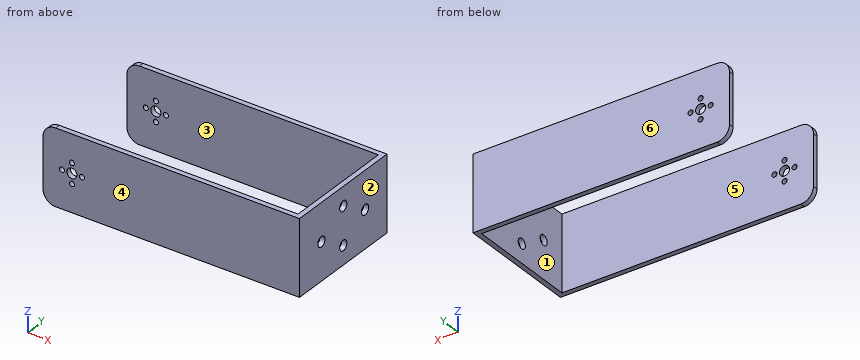
from build123d import *

# Parameters (mm, degrees)
EKSTR_ZYON_NCE1_DEPTH = 60
RADYUS1_R             = 10
KES_EKSTR_ZYON1_REACH = 236.137
IZIM2_R               = 4
IZIM2_R_2             = 2
KES_EKSTR_ZYON2_REACH = 234.491
IZIM3_R               = 4


with BuildPart() as part:
    # izim1 → Ekstr_zyon-_nce1 (new body)
    with BuildSketch(Plane.XY):
        Polygon((0, 0), (200, 0), (200, 90), (0, 90), (0, 94), (204, 94), (204, -4), (0, -4), align=None)
    extrude(amount=EKSTR_ZYON_NCE1_DEPTH)

    # Radyus1
    radyus1_edges = [part.edges().sort_by_distance(p)[0] for p in [
        (0, -2, 60),
        (0, 92, 60),
        (0, -2, 0),
        (0, 92, 0),
    ]]
    fillet(radyus1_edges, radius=RADYUS1_R)

    # izim2 → Kes-Ekstr_zyon1 (cut, up to next)
    with BuildSketch(Plane(origin=(0, 94, 0), x_dir=(1, 0, 0), z_dir=(0, 1, 0)), mode=Mode.PRIVATE) as kes_ekstr_zyon1_sk1:
        with Locations(Location((23, -30, 0), (0, 0, 270))):
            Circle(IZIM2_R)
    kes_ekstr_zyon1_tool1 = extrude(kes_ekstr_zyon1_sk1.sketch, amount=-KES_EKSTR_ZYON1_REACH, mode=Mode.PRIVATE) & part.part
    # izim2 → Kes-Ekstr_zyon1 (cut, up to next)
    with BuildSketch(Plane(origin=(0, 94, 0), x_dir=(1, 0, 0), z_dir=(0, 1, 0)), mode=Mode.PRIVATE) as kes_ekstr_zyon1_sk2:
        with Locations(Location((23, -22, 0), (0, 0, 270))):
            Circle(IZIM2_R_2)
    kes_ekstr_zyon1_tool2 = extrude(kes_ekstr_zyon1_sk2.sketch, amount=-KES_EKSTR_ZYON1_REACH, mode=Mode.PRIVATE) & part.part
    # izim2 → Kes-Ekstr_zyon1 (cut, up to next)
    with BuildSketch(Plane(origin=(0, 94, 0), x_dir=(1, 0, 0), z_dir=(0, 1, 0)), mode=Mode.PRIVATE) as kes_ekstr_zyon1_sk3:
        with Locations(Location((23, -38, 0), (0, 0, 270))):
            Circle(IZIM2_R_2)
    kes_ekstr_zyon1_tool3 = extrude(kes_ekstr_zyon1_sk3.sketch, amount=-KES_EKSTR_ZYON1_REACH, mode=Mode.PRIVATE) & part.part
    # izim2 → Kes-Ekstr_zyon1 (cut, up to next)
    with BuildSketch(Plane(origin=(0, 94, 0), x_dir=(1, 0, 0), z_dir=(0, 1, 0)), mode=Mode.PRIVATE) as kes_ekstr_zyon1_sk4:
        with Locations(Location((31, -30, 0), (0, 0, 270))):
            Circle(IZIM2_R_2)
    kes_ekstr_zyon1_tool4 = extrude(kes_ekstr_zyon1_sk4.sketch, amount=-KES_EKSTR_ZYON1_REACH, mode=Mode.PRIVATE) & part.part
    # izim2 → Kes-Ekstr_zyon1 (cut, up to next)
    with BuildSketch(Plane(origin=(0, 94, 0), x_dir=(1, 0, 0), z_dir=(0, 1, 0)), mode=Mode.PRIVATE) as kes_ekstr_zyon1_sk5:
        with Locations(Location((15, -30, 0), (0, 0, 270))):
            Circle(IZIM2_R_2)
    kes_ekstr_zyon1_tool5 = extrude(kes_ekstr_zyon1_sk5.sketch, amount=-KES_EKSTR_ZYON1_REACH, mode=Mode.PRIVATE) & part.part
    kes_ekstr_zyon1_1 = kes_ekstr_zyon1_tool1.solids().sort_by_distance((23, 94, 30))[0]
    add(kes_ekstr_zyon1_1, mode=Mode.SUBTRACT)
    kes_ekstr_zyon1_2 = kes_ekstr_zyon1_tool2.solids().sort_by_distance((23, 94, 22))[0]
    add(kes_ekstr_zyon1_2, mode=Mode.SUBTRACT)
    kes_ekstr_zyon1_3 = kes_ekstr_zyon1_tool3.solids().sort_by_distance((23, 94, 38))[0]
    add(kes_ekstr_zyon1_3, mode=Mode.SUBTRACT)
    kes_ekstr_zyon1_4 = kes_ekstr_zyon1_tool4.solids().sort_by_distance((31, 94, 30))[0]
    add(kes_ekstr_zyon1_4, mode=Mode.SUBTRACT)
    kes_ekstr_zyon1_5 = kes_ekstr_zyon1_tool5.solids().sort_by_distance((15, 94, 30))[0]
    add(kes_ekstr_zyon1_5, mode=Mode.SUBTRACT)
    kes_ekstr_zyon1 = kes_ekstr_zyon1_1 + kes_ekstr_zyon1_2 + kes_ekstr_zyon1_3 + kes_ekstr_zyon1_4 + kes_ekstr_zyon1_5  # Kes-Ekstr_zyon1 as one shape, for the pattern or mirror that repeats it

    # Aynalama1: Kes-Ekstr_zyon1 across plane
    add(kes_ekstr_zyon1.mirror(Plane.ZX.offset(45)), mode=Mode.SUBTRACT)

    # izim3 → Kes-Ekstr_zyon2 (cut, up to next)
    with BuildSketch(Plane(origin=(204, 0, 0), x_dir=(0, 0, -1), z_dir=(1, 0, 0)), mode=Mode.PRIVATE) as kes_ekstr_zyon2_sk1:
        with Locations((-30, 69.5)):
            Circle(IZIM3_R)
    kes_ekstr_zyon2_tool1 = extrude(kes_ekstr_zyon2_sk1.sketch, amount=-KES_EKSTR_ZYON2_REACH, mode=Mode.PRIVATE) & part.part
    # izim3 → Kes-Ekstr_zyon2 (cut, up to next)
    with BuildSketch(Plane(origin=(204, 0, 0), x_dir=(0, 0, -1), z_dir=(1, 0, 0)), mode=Mode.PRIVATE) as kes_ekstr_zyon2_sk2:
        with Locations((-45, 45)):
            Circle(IZIM3_R)
    kes_ekstr_zyon2_tool2 = extrude(kes_ekstr_zyon2_sk2.sketch, amount=-KES_EKSTR_ZYON2_REACH, mode=Mode.PRIVATE) & part.part
    # izim3 → Kes-Ekstr_zyon2 (cut, up to next)
    with BuildSketch(Plane(origin=(204, 0, 0), x_dir=(0, 0, -1), z_dir=(1, 0, 0)), mode=Mode.PRIVATE) as kes_ekstr_zyon2_sk3:
        with Locations(Location((-15, 45, 0), (0, 0, 180))):
            Circle(IZIM3_R)
    kes_ekstr_zyon2_tool3 = extrude(kes_ekstr_zyon2_sk3.sketch, amount=-KES_EKSTR_ZYON2_REACH, mode=Mode.PRIVATE) & part.part
    # izim3 → Kes-Ekstr_zyon2 (cut, up to next)
    with BuildSketch(Plane(origin=(204, 0, 0), x_dir=(0, 0, -1), z_dir=(1, 0, 0)), mode=Mode.PRIVATE) as kes_ekstr_zyon2_sk4:
        with Locations(Location((-30, 20.5, 0), (0, 0, 180))):
            Circle(IZIM3_R)
    kes_ekstr_zyon2_tool4 = extrude(kes_ekstr_zyon2_sk4.sketch, amount=-KES_EKSTR_ZYON2_REACH, mode=Mode.PRIVATE) & part.part
    add(kes_ekstr_zyon2_tool1.solids().sort_by_distance((204, 69.5, 30))[0], mode=Mode.SUBTRACT)
    add(kes_ekstr_zyon2_tool2.solids().sort_by_distance((204, 45, 45))[0], mode=Mode.SUBTRACT)
    add(kes_ekstr_zyon2_tool3.solids().sort_by_distance((204, 45, 15))[0], mode=Mode.SUBTRACT)
    add(kes_ekstr_zyon2_tool4.solids().sort_by_distance((204, 20.5, 30))[0], mode=Mode.SUBTRACT)


solid = part.part
Build history of the part. All positions in model axes, mm. Face numbers are marked on the shaded views. A direction names the side the tool comes from. Round coordinates to 2 decimals unless told otherwise and drop trailing zeros. Loops run counter-clockwise (first coordinate to the right, second up) from the corner with the lowest first, then second, coordinate; pieces in that order, holes last. Notation, with made-up numbers: (49.25, 4) -> (60.25, 4) arc R23 cw to (60.25, 13) -> close; hole circle Ø4 at (51.5, -30). An arc over 180 degrees is marked (long way). One line per item, written item: value. Start each with the question number.
Q1. Cut at A-A on z = 38. List the corners of the cut face in (x, y).
Q2. 3-axis set-ups, long thin cutter, end or side, ignore diameter. For the marked faces 1 and 2: which of +Z, -Z, +X, -X, +Y, -Y reach the whole face in a straight line?
Q3. Drop flat-ended pins along their axis: pin 1 Ø5 at (x, z) = (23, 38) entering from -Y; pin 2 Ø12 at (x, y) = (79, 7.5) entering from -Z; pin 3 Ø2 at (y, z) = (73.5, 46) entering from -X. Give the stop position or say it passes through.
Q4. Cut at B-B on x = 31. List the corners of the cut face in (y, z).
Q5. Probe line 1 along Y through (x, z) = (202.05, 30); line 2 along Y through (x, z) = (38, 52); line 3 along X through (y, z) = (-1.25, 22). List the from-to ranges inside material, lowest first.
Q6. Cut at C-C on y = 69.5. List the corners of the cut face in (x, z).
Q7. Cut at D-D on x = 70. List the corners of the cut face in (y, z).
Q8. Two-plate mould, pull along Y, no slides. Class the marked faces 3, 4, 5 and 6: released by +Y, released by -Y, zero draft, split by the parting line, or undercut.
Computed:
1. outline: (0, -4) -> (21, -4) -> (21, 0) -> (0, 0) -> close; (0, 90) -> (21, 90) -> (21, 94) -> (0, 94) -> close; (25, -4) -> (204, -4) -> (204, 94) -> (25, 94) -> (25, 90) -> (200, 90) -> (200, 0) -> (25, 0) -> close
2. face 1: +Z, -Z, -X
2. face 2: +Z, -Z, +X, +Y, -Y
3. pin 1: y = -4
3. pin 2: through
3. pin 3: x = 200
4. outline: (-4, 0) -> (0, 0) -> (0, 28) -> (-4, 28) -> close; (-4, 32) -> (0, 32) -> (0, 60) -> (-4, 60) -> close; (90, 0) -> (94, 0) -> (94, 28) -> (90, 28) -> close; (90, 32) -> (94, 32) -> (94, 60) -> (90, 60) -> close
5. line 1: -4 to 16.5, 24.5 to 65.5, 73.5 to 94
5. line 2: -4 to 0, 90 to 94
5. line 3: 0 to 21, 25 to 204
6. outline: (200, 0) -> (204, 0) -> (204, 26) -> (200, 26) -> close; (200, 34) -> (204, 34) -> (204, 60) -> (200, 60) -> close
7. outline: (-4, 0) -> (0, 0) -> (0, 60) -> (-4, 60) -> close; (90, 0) -> (94, 0) -> (94, 60) -> (90, 60) -> close
8. face 3: undercut
8. face 4: released by -Y
8. face 5: undercut
8. face 6: released by +Y
